from build123d import *

# Parameters (mm, degrees)
SKETCH3_R           = 35
SKETCH3_R_2         = 32
BOSS_EXTRUDE1_DEPTH = 68
SKETCH4_R           = 12.25
CUT_EXTRUDE1_DEPTH  = 85.107074613
SKETCH5_R           = 12.25
CUT_EXTRUDE2_DEPTH  = 85.107074777


with BuildPart() as part:
    # Sketch3 → Boss-Extrude1 (new, symmetric)
    with BuildSketch(Plane(origin=(0, 0, 0), x_dir=(0, 0, -1), z_dir=(1, 0, 0))):
        Circle(SKETCH3_R)
        Circle(SKETCH3_R_2, mode=Mode.SUBTRACT)
    extrude(amount=BOSS_EXTRUDE1_DEPTH, both=True)

    # Sketch4 → Cut-Extrude1 (cut, through all)
    with BuildSketch(Plane(origin=(0, 0, 0), x_dir=(1, 0, 0), z_dir=(0, 1, 0))):
        with Locations(Location((-41.5, 0, 0), (0, 0, 270))):
            Circle(SKETCH4_R)
    extrude(amount=-CUT_EXTRUDE1_DEPTH, mode=Mode.SUBTRACT)

    # Sketch5 → Cut-Extrude2 (cut, through all)
    with BuildSketch(Plane(origin=(0, 0, 0), x_dir=(1, 0, 0), z_dir=(0, 1, 0))):
        with Locations(Location((41.5, 0, 0), (0, 0, 90))):
            Circle(SKETCH5_R)
    extrude(amount=CUT_EXTRUDE2_DEPTH, mode=Mode.SUBTRACT)


solid = part.part
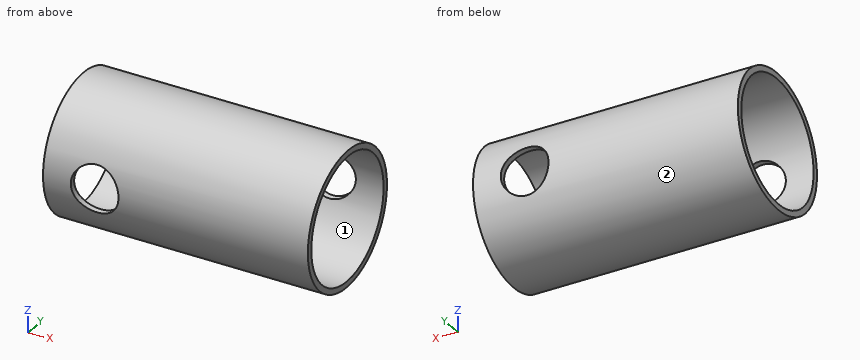
Source: CAD feature listing. Evaluate the final solid. Frame: model axes, mm. Face numbers are marked on the shaded views. Round coordinates to 2 decimals unless told otherwise and drop trailing zeros. Order: outer loops, then holes, each group sorted by start corner. A loop starts at its lowest first (then second) coordinate and runs counter-clockwise, first axis right, second up. Notation, with made-up numbers: (79, -18.75) - (129, -18.75) arc R22 cw to (129, -4.75) - close; hole circle Ø3 at (89.5, 0). An arc over 180 degrees is marked (long way). Use a Markdown table: item, result. Add a question column.
1. Line query: probe 1 along Z at (x, y) = (32, 0.5); probe 2 along Y at (x, z) = (40, 25.5); probe 3 along Z at (x, y) = (41, 31). Output: solid intervals per line, ascending.
2. Section query C-C (z = 18). Return the cut outline in (x, y).
3. First-contact query: pin 1 (1 mm diameter, centred on x = -43.5, y = 10, fed in from -Z); pin 2 (10 mm diameter, centred on y = -3.5, z = -26, fed in from -X); pin 3 (6 mm diameter, centred on x = 23, z = -15, fed in from -Y); pin 4 (4 mm diameter, centred on x = 32.5, z = 25, fed in from +Y). Flat tips, straight axial feed; report the tip coordinate or a pass-through.
4. Section query A-A (z = 0). Return the cut outline in (x, y).
5. Section query B-B (y = -2.5). Return the cut outline in (x, z).
6. Section query D-D (x = -9). Return the cut outline in (y, z), then the cut area to 3 significant figures.
7. Mould query, pull axis Z, two halves, no side actions, for the marked faces 1 and 2. Classes: +Z half, -Z half, draft (parallel to the pull), parting line (faces both ways), or undercut.
Derived:
| question | item | result |
|---|---|---|
| 1 | probe 1 | -35 to -32, 32 to 35 |
| 1 | probe 2 | -23.97 to -19.33, 19.33 to 23.97 |
| 1 | probe 3 | -16.25 to -12.24, 12.24 to 16.25 |
| 2 | outline | (-68, -30.02) - (68, -30.02) - (68, -26.46) - (-68, -26.46) - close; (-68, 26.46) - (68, 26.46) - (68, 30.02) - (-68, 30.02) - close |
| 3 | pin 1 | z = -33.69 |
| 3 | pin 2 | through |
| 3 | pin 3 | y = -32.88 |
| 3 | pin 4 | y = 26.38 |
| 4 | outline | (-68, -35) - (-53.75, -35) - (-53.75, -32) - (-68, -32) - close; (-68, 32) - (29.25, 32) - (29.25, 35) - (-68, 35) - close; (-29.25, -35) - (68, -35) - (68, -32) - (-29.25, -32) - close; (53.75, 32) - (68, 32) - (68, 35) - (53.75, 35) - close |
| 5 | outline | (-68, -34.91) - (68, -34.91) - (68, -31.9) - (-68, -31.9) - close; (-68, 31.9) - (68, 31.9) - (68, 34.91) - (-68, 34.91) - close |
| 6 | outline | circle Ø70 at (0, 0); hole circle Ø64 at (0, 0) |
| 6 | area | 631 mm2 |
| 7 | face 1 | undercut |
| 7 | face 2 | parting line |
